```python
from build123d import *

# Parameters (mm, degrees)
SKETCH1_W           = 17
SKETCH1_H           = 6
BOSS_EXTRUDE1_DEPTH = 43
SKETCH3_W           = 17.0508
SKETCH3_H           = 6.0508
BOSS_EXTRUDE2_DEPTH = 6.35
SKETCH4_R           = 0.635
BOSS_EXTRUDE4_DEPTH = 1.5875


with BuildPart() as part:
    # Sketch1 → Boss-Extrude1 (new body)
    with BuildSketch(Plane.XY):
        with Locations((8.5, 3)):
            Rectangle(SKETCH1_W, SKETCH1_H)
    extrude(amount=BOSS_EXTRUDE1_DEPTH)

    # Sketch3 → Boss-Extrude2 (add)
    with BuildSketch(Plane.XY.offset(43)):
        with Locations((8.5, 3)):
            Rectangle(SKETCH3_W, SKETCH3_H)
    extrude(amount=-BOSS_EXTRUDE2_DEPTH)

    # Sketch4 → Boss-Extrude4 (add)
    with BuildSketch(Plane(origin=(17, 0, 0), x_dir=(0, 0, -1), z_dir=(1, 0, 0))):
        with Locations(Location((-42.193767819, 1.041160234, 0), (0, 0, 90))):
            Circle(SKETCH4_R)
        with Locations(Location((-42.193767819, 2.438160234, 0), (0, 0, 90))):
            Circle(SKETCH4_R)
    extrude(amount=BOSS_EXTRUDE4_DEPTH)


solid = part.part
```
The listing builds one solid part. Answer for the finished solid, in the listing's coordinates (mm). A direction names the side the tool comes from. Round coordinates to 2 decimals unless told otherwise and drop trailing zeros. Order: outer loops, then holes, each group sorted by start corner. A loop starts at its lowest first (then second) coordinate and runs counter-clockwise, first axis right, second up. Notation, with made-up numbers: (72, 25.25) - (78, 25.25) arc R29 cw to (78, 46.25) - close; hole circle Ø9 at (-27, 41). An arc over 180 degrees is marked (long way). Put each result on its own line as item: value. Start each with the question number.
(1) Determine the mould class of faces 4 (the flat face through (8, 6.025, 40)), 5 (the cylindrical face through (17.796, 2.301, 41.574)), 6 (the flat face through (8, -0.025, 40)) for opening direction Y: released by +Y, released by -Y, zero draft, split by the parting line, or undercut.
(2) Straight lines are drawn through the part: probe 1 along X at (y, z) = (2.75, 17); probe 2 along Y at (x, z) = (10.5, 2); probe 3 along Z at (x, y) = (17.75, 1). For each, find the intervals that lie inside material, in ascending order. Write a range as from..to.
(3) Find section B-B (z = 35.5). Give the vertices of the cut face in (x, y).
(4) For faces 1 (the flat face through (17, 3, 18)), 2 (the cylindrical face through (17.796, 0.904, 41.574)), 3 (the flat face through (18.588, 1, 42)), determine the directions among +Z, -Z, +X, -X, +Y, -Y from which every point of the face is accessible in a straight line to the end or side of a thin tool.
(5) Given P1, Ø8.5, axis at x = 10.5, z = 27, coming from the +Y side; P2, Ø3, axis at y = 4.5, z = 40, coming from the +X side; P3, Ø5, axis at x = 4.5, z = 21.5, coming from the -Y side, each flat-ended and moving along its own axis, determine where each tip first touches the part or whether it passes through.
Reply:
1. face 4: released by +Y
1. face 5: undercut
1. face 6: released by -Y
2. probe 1: 0..17
2. probe 2: 0..6
2. probe 3: 41.56..42.83
3. outline: (0, 0) - (17, 0) - (17, 6) - (0, 6) - close
4. face 1: -Z, +X, +Y, -Y
4. face 2: +X
4. face 3: +Z, -Z, +X, +Y, -Y
5. P1: y = 6
5. P2: x = 17.03
5. P3: y = 0
